Geometry: final body of the model. Coordinates: model frame, mm. Round coordinates to 2 decimals unless told otherwise and drop trailing zeros. Write each loop counter-clockwise with the first axis right and the second up, starting at its lowest first coordinate (ties: lowest second). Pieces come first, ordered by that corner, then holes. Notation, with made-up numbers: (25, -28.5) -> (56, -28.5) arc R26 cw to (56, -5.5) -> close; hole circle Ø3 at (17.25, 29). An arc over 180 degrees is marked (long way). Use one line per item in the form item = value. Start each with the question number.
1. Cut plane A-A, the plane x = -10. Return the cut outline in (y, z), plus the area to 3 significant figures.
2. Cut plane C-C, the plane x = -36. Return the cut outline in (y, z).
3. Cut plane D-D, the plane x = 0. Return the cut outline in (y, z), plus the area to 3 significant figures.
4. Line query: L1, parallel to Y at x = -43, z = 0; L2, parallel to X at y = 4.5, z = -1.8; L3, parallel to X at y = -13, z = 1.9. Output: solid intervals per line, ascending.
5. Cut plane B-B, the plane y = 2.5. Return the cut outline in (x, z).
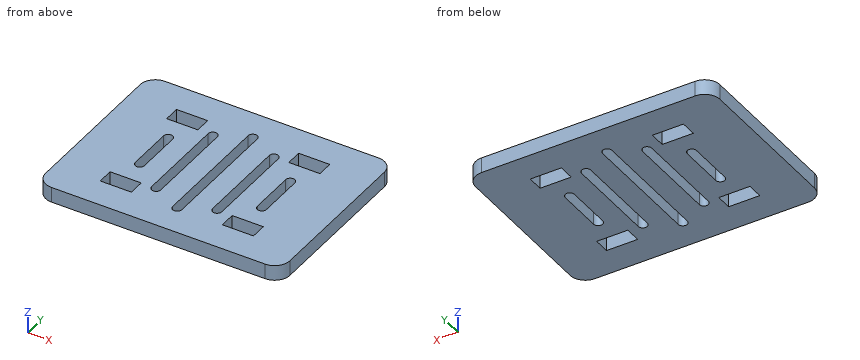
```python
from build123d import *

# Parameters (mm, degrees)
SKETCH1_W           = 5.2
SKETCH1_H           = 10.2
BOSS_EXTRUDE1_DEPTH = 2.5
FILLET1_R           = 5


with BuildPart() as part:
    # Sketch1 → Boss-Extrude1 (new, symmetric)
    with BuildSketch(Plane(origin=(0, 0, 0), x_dir=(0, 1, 0), z_dir=(0, 0, 1))):
        Polygon((30, 0), (30, -20), (-30, -20), (-30, 0), (-30, 40), (-30, 60), (30, 60), (30, 40), align=None)
        with Locations((17.6, 0)):
            Rectangle(SKETCH1_W, SKETCH1_H, mode=Mode.SUBTRACT)
        with Locations((17.6, 40)):
            Rectangle(SKETCH1_W, SKETCH1_H, mode=Mode.SUBTRACT)
        with Locations((-17.6, 0)):
            Rectangle(SKETCH1_W, SKETCH1_H, mode=Mode.SUBTRACT)
        with Locations((-17.6, 40)):
            Rectangle(SKETCH1_W, SKETCH1_H, mode=Mode.SUBTRACT)
        with BuildLine():
            Line((7.5, 41.5), (-7.5, 41.5))
            ThreePointArc((-7.5, 41.5), (-9, 40), (-7.5, 38.5))
            Line((-7.5, 38.5), (7.5, 38.5))
            ThreePointArc((7.5, 38.5), (9, 40), (7.5, 41.5))
        make_face(mode=Mode.SUBTRACT)
        with BuildLine():
            Line((15, 31.5), (-15, 31.5))
            ThreePointArc((-15, 31.5), (-16.5, 30), (-15, 28.5))
            Line((-15, 28.5), (15, 28.5))
            ThreePointArc((15, 28.5), (16.5, 30), (15, 31.5))
        make_face(mode=Mode.SUBTRACT)
        with BuildLine():
            Line((20, 21.5), (-20, 21.5))
            ThreePointArc((-20, 21.5), (-21.5, 20), (-20, 18.5))
            Line((-20, 18.5), (20, 18.5))
            ThreePointArc((20, 18.5), (21.5, 20), (20, 21.5))
        make_face(mode=Mode.SUBTRACT)
        with BuildLine():
            Line((15, 11.5), (-15, 11.5))
            ThreePointArc((-15, 11.5), (-16.5, 10), (-15, 8.5))
            Line((-15, 8.5), (15, 8.5))
            ThreePointArc((15, 8.5), (16.5, 10), (15, 11.5))
        make_face(mode=Mode.SUBTRACT)
        with BuildLine():
            Line((7.5, 1.5), (-7.5, 1.5))
            ThreePointArc((-7.5, 1.5), (-9, 0), (-7.5, -1.5))
            Line((-7.5, -1.5), (7.5, -1.5))
            ThreePointArc((7.5, -1.5), (9, 0), (7.5, 1.5))
        make_face(mode=Mode.SUBTRACT)
    extrude(amount=BOSS_EXTRUDE1_DEPTH, both=True)

    # Fillet1
    fillet1_edges = [part.edges().sort_by_distance(p)[0] for p in [
        (-60, -30, 0),
        (-60, 30, 0),
        (20, 30, 0),
        (20, -30, 0),
    ]]
    fillet(fillet1_edges, radius=FILLET1_R)


solid = part.part
```
Outcome:
q1.outline = (-30, -2.5) -> (-16.5, -2.5) -> (-16.5, 2.5) -> (-30, 2.5) -> close; (16.5, -2.5) -> (30, -2.5) -> (30, 2.5) -> (16.5, 2.5) -> close
q1.area = 135 mm^2
q2.outline = (-30, -2.5) -> (-20.2, -2.5) -> (-20.2, 2.5) -> (-30, 2.5) -> close; (-15, -2.5) -> (15, -2.5) -> (15, 2.5) -> (-15, 2.5) -> close; (20.2, -2.5) -> (30, -2.5) -> (30, 2.5) -> (20.2, 2.5) -> close
q3.outline = (-30, -2.5) -> (-20.2, -2.5) -> (-20.2, 2.5) -> (-30, 2.5) -> close; (-15, -2.5) -> (-9, -2.5) -> (-9, 2.5) -> (-15, 2.5) -> close; (9, -2.5) -> (15, -2.5) -> (15, 2.5) -> (9, 2.5) -> close; (20.2, -2.5) -> (30, -2.5) -> (30, 2.5) -> (20.2, 2.5) -> close
q3.area = 158 mm^2
q4.L1 = -30 to -20.2, -15 to 15, 20.2 to 30
q4.L2 = -60 to -41.5, -38.5 to -31.5, -28.5 to -21.5, -18.5 to -11.5, -8.5 to -1.5, 1.5 to 20
q4.L3 = -60 to -31.5, -28.5 to -21.5, -18.5 to -11.5, -8.5 to 20
q5.outline = (-60, -2.5) -> (-41.5, -2.5) -> (-41.5, 2.5) -> (-60, 2.5) -> close; (-38.5, -2.5) -> (-31.5, -2.5) -> (-31.5, 2.5) -> (-38.5, 2.5) -> close; (-28.5, -2.5) -> (-21.5, -2.5) -> (-21.5, 2.5) -> (-28.5, 2.5) -> close; (-18.5, -2.5) -> (-11.5, -2.5) -> (-11.5, 2.5) -> (-18.5, 2.5) -> close; (-8.5, -2.5) -> (-1.5, -2.5) -> (-1.5, 2.5) -> (-8.5, 2.5) -> close; (1.5, -2.5) -> (20, -2.5) -> (20, 2.5) -> (1.5, 2.5) -> close
